The listing builds one solid part. Answer for the finished solid, in the listing's coordinates (mm). A direction names the side the tool comes from. Round coordinates to 2 decimals unless told otherwise and drop trailing zeros. Order: outer loops, then holes, each group sorted by start corner. A loop starts at its lowest first (then second) coordinate and runs counter-clockwise, first axis right, second up. Notation, with made-up numbers: (-13.5, 3) -> (26.5, 3) arc R17 ccw to (26.5, 33) -> close; hole circle Ø5 at (-35.5, 21.25). An arc over 180 degrees is marked (long way). Return JSON: item names as keys, results as strings. Group by question number.
(1) The part is cut by section C-C (y = -7.5). Determine the outline of the cut face in (x, z), plus the area to 3 significant figures.
(2) Determine the mould class of faces 1 (the face through (-11, 0, -3)), 2 (the face through (7.177, 7.952, -1.479)), 3 (the face through (-9.88, -1.76, -1.48)) for opening direction X: +X half, -X half, draft (parallel to the pull), parting line (faces both ways), or undercut.
(3) The part is cut by section D-D (y = 33). Determine the outline of the cut face in (x, z), plus the area to 3 significant figures.
(4) The part is cut by section A-A (z = -0.8). Determine the outline of the cut face in (x, y) (3 decimals), plus the area to 3 significant figures.
(5) Consider line 1 (Y direction, x = 0.5, z = 0.2); line 2 (Y direction, x = -7, z = -1.55); line 3 (Z direction, x = -1, y = -5). Determine where each line is inside the solid, lowest interval first. Write a range as [from, to].
(6) Which of the six approach directions +Z, -Z, +X, -X, +Y, -Y give full straight-line access (tool end or side, diameter ignored) to faces 4 (the face through (-6.391, 7.647, -1.479)), 5 (the face through (9.88, -1.76, -1.48)), 6 (the face through (6.463, -7.675, -1.479))?
(7) The part is cut by section B-B (y = 7.5). Determine the outline of the cut face in (x, z).
(8) Each of these flat-tipped pins is pushed along its axis until it touches: pin 1 (2 mm diameter, centred on y = 23, z = -0.5, fed in from -X); pin 2 (2.5 mm diameter, centred on x = 6.5, y = -3.75, fed in from +Z); pin 3 (5.5 mm diameter, centred on x = 0, y = 0, fed in from -Z); pin 4 (1 mm diameter, centred on y = 32, z = -1.5, fed in from +X). Where does it stop, or does it pass through?
from build123d import *

# Parameters (mm, degrees)
SKETCH_1_R      = 1.7
SKETCH_1_R_2    = 1.75
SKETCH_1_R_3    = 1.5
EXTRUDE_1_DEPTH = 2
SKETCH_2_R      = 1.7
EXTRUDE_2_DEPTH = 3


with BuildPart() as part:
    # 草图1 → 凸台-拉伸1 (new body)
    with BuildSketch(Plane.XY):
        with BuildLine():
            Line((4.943429983, 50.75), (12.358574958, 1.875))
            ThreePointArc((12.358574958, 1.875), (-3.784680756, -11.913277953), (-9.010584258, 8.663681166))
            ThreePointArc((-9.010584258, 8.663681166), (-0.173058011, 27.293788413), (-4.325142467, 47.491386311))
            ThreePointArc((-4.325142467, 47.491386311), (-1.658375909, 54.716968236), (4.943429983, 50.75))
        make_face()
        with Locations((0, 50)):
            Circle(SKETCH_1_R, mode=Mode.SUBTRACT)
        Circle(SKETCH_1_R_2, mode=Mode.SUBTRACT)
        with Locations((-6.495190528, -3.75)):
            Circle(SKETCH_1_R_3, mode=Mode.SUBTRACT)
        with Locations((-6.495190528, 3.75)):
            Circle(SKETCH_1_R_3, mode=Mode.SUBTRACT)
        with Locations((0, 7.5)):
            Circle(SKETCH_1_R_3, mode=Mode.SUBTRACT)
        with Locations((6.495190528, 3.75)):
            Circle(SKETCH_1_R_3, mode=Mode.SUBTRACT)
        with Locations((6.495190528, -3.75)):
            Circle(SKETCH_1_R_3, mode=Mode.SUBTRACT)
        with Locations((0, -7.5)):
            Circle(SKETCH_1_R_3, mode=Mode.SUBTRACT)
    extrude(amount=EXTRUDE_1_DEPTH)

    # 草图2 → 凸台-拉伸2 (add)
    with BuildSketch(Plane(origin=(0, 0, 0), x_dir=(-1, 0, 0), z_dir=(0, 0, -1))):
        with BuildLine():
            Line((-12.104606684, 3.548965842), (-12.358574958, 1.875))
            ThreePointArc((-12.358574958, 1.875), (-12.473254326, -0.817267717), (-12.008260108, -3.471554287))
            Line((-12.008260108, -3.471554287), (-7.687556684, 0))
            Line((-7.687556684, 0), (-12.104606684, 3.548965842))
        make_face()
        with BuildLine():
            Line((-4.943429983, 50.75), (-11.218143605, 9.391856725))
            ThreePointArc((-11.218143605, 9.391856725), (-10.811437733, 9.330472298), (-10.418112816, 9.210167583))
            Line((-10.418112816, 9.210167583), (-3.843778342, 6.657619381))
            Line((-3.843778342, 6.657619381), (-2.767182691, 13.62743415))
            ThreePointArc((-2.767182691, 13.62743415), (0, 16), (2.767182691, 13.62743415))
            Line((2.767182691, 13.62743415), (3.843778342, 6.657619381))
            Line((3.843778342, 6.657619381), (9.010584258, 8.663681166))
            ThreePointArc((9.010584258, 8.663681166), (0.173058011, 27.293788413), (4.325142467, 47.491386311))
            ThreePointArc((4.325142467, 47.491386311), (1.658375909, 54.716968236), (-4.943429983, 50.75))
        make_face()
        with Locations((0, 50)):
            Circle(SKETCH_2_R, mode=Mode.SUBTRACT)
        with BuildLine():
            Line((7.687556684, 0), (12.008260108, 3.471554287))
            ThreePointArc((12.008260108, 3.471554287), (12.5, 0), (12.008260108, -3.471554287))
            Line((12.008260108, -3.471554287), (7.687556684, 0))
        make_face()
        with BuildLine():
            Line((3.843778342, -6.657619381), (9.010584258, -8.663681166))
            ThreePointArc((9.010584258, -8.663681166), (6.25, -10.825317547), (2.997675851, -12.135235453))
            Line((2.997675851, -12.135235453), (3.843778342, -6.657619381))
        make_face()
        with BuildLine():
            Line((-3.843778342, -6.657619381), (-2.997675851, -12.135235453))
            ThreePointArc((-2.997675851, -12.135235453), (-6.25, -10.825317547), (-9.010584258, -8.663681166))
            Line((-9.010584258, -8.663681166), (-3.843778342, -6.657619381))
        make_face()
    extrude(amount=EXTRUDE_2_DEPTH)


solid = part.part
Answer below:
{
 "1": {"outline": "(-10, 0) -> (-6.01, 0) -> (-6.01, -3) -> (-3.71, -3) -> (-3.71, 0) -> (-1.5, 0) -> (-1.5, 2) -> (-10, 2) -> close; (1.5, 0) -> (3.71, 0) -> (3.71, -3) -> (6.01, -3) -> (6.01, 0) -> (10, 0) -> (10, 2) -> (1.5, 2) -> close", "area": "47.8 mm²"},
 "2": {"face 1": "draft", "face 2": "+X half", "face 3": "undercut"},
 "3": {"outline": "(0.01, -3) -> (7.64, -3) -> (7.64, 2) -> (0.01, 2) -> close", "area": "38.1 mm²"},
 "4": {"outline": "(-12.008, -3.472) -> (-7.688, 0) -> (-12.008, 3.472) arc R12.5 ccw to start; (-9.011, -8.664) arc R12.5 ccw to (-2.998, -12.135) -> (-3.844, -6.658) -> close; (-9.011, 8.664) -> (-3.844, 6.658) -> (-2.767, 13.627) arc R2.8 cw to (2.767, 13.627) -> (3.844, 6.658) -> (10.418, 9.21) arc R2.8 cw to (11.218, 9.392) -> (4.943, 50.75) arc R5 ccw (long way) to (-4.325, 47.491) arc R32.497 cw to start; (2.998, -12.135) arc R12.5 ccw to (9.011, -8.664) -> (3.844, -6.658) -> close; (7.688, 0) -> (12.008, -3.472) arc R12.5 ccw to (12.359, 1.875) -> (12.105, 3.549) -> close; hole circle Ø3.4 at (0, 50)", "area": "503 mm²"},
 "5": {"line 1": "y = [-12.49, -8.91], [-6.09, -1.68], [1.68, 6.09], [8.91, 48.38], [51.62, 54.97]", "line 2": "y = [-10.36, -7.88], [7.88, 10.96]", "line 3": "z = [0, 2]"},
 "6": {"face 4": "-Z, -X", "face 5": "-Z", "face 6": "-Z, +X"},
 "7": {"outline": "(-10, 0) -> (-6.01, 0) -> (-6.01, -3) -> (-3.71, -3) -> (-3.71, 0) -> (-1.5, 0) -> (-1.5, 2) -> (-10, 2) -> close; (1.5, 0) -> (3.71, 0) -> (3.71, -3) -> (6.01, -3) -> (6.01, 0) -> (11.51, 0) -> (11.51, 2) -> (1.5, 2) -> close"},
 "8": {"pin 1": "stops at x = -1.26", "pin 2": "passes through", "pin 3": "stops at z = 0", "pin 4": "stops at x = 7.86"}
}
